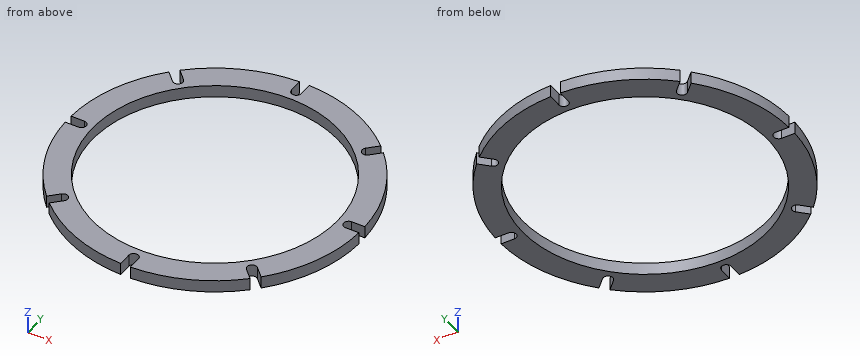
```python
from build123d import *

# Parameters (mm, degrees)
SKETCH1_R           = 121.15
SKETCH1_R_2         = 101.15
BOSS_EXTRUDE1_DEPTH = 10
CUT_EXTRUDE1_DEPTH  = 10
CIRPATTERN1_COUNT   = 8


with BuildPart() as part:
    # Sketch1 → Boss-Extrude1 (new body)
    with BuildSketch(Plane.XY):
        Circle(SKETCH1_R)
        Circle(SKETCH1_R_2, mode=Mode.SUBTRACT)
    extrude(amount=BOSS_EXTRUDE1_DEPTH)

    # Sketch2 → Cut-Extrude1 (cut)
    with BuildSketch(Plane.XY):
        with BuildLine():
            Line((-4, 110.15), (-4, 123.851971246))
            Line((-4, 123.851971246), (4, 123.851971246))
            Line((4, 123.851971246), (4, 110.15))
            ThreePointArc((4, 110.15), (0, 106.15), (-4, 110.15))
        make_face()
    cut_extrude1 = extrude(amount=CUT_EXTRUDE1_DEPTH, mode=Mode.SUBTRACT)

    # CirPattern1: Cut-Extrude1 ×8 about axis
    cirpattern1_axis = Axis((0, 0, 0), (0, 0, 1))
    for i in range(1, CIRPATTERN1_COUNT):
        add(cut_extrude1.rotate(cirpattern1_axis, i * 360 / CIRPATTERN1_COUNT), mode=Mode.SUBTRACT)


solid = part.part
```
Geometry check sheet. Reference: the model listing, model coordinates, mm. Give positions to 0.01 mm unless a question says otherwise; leave off trailing zeros. Write each loop counter-clockwise with the first axis right and the second up, starting at its lowest first coordinate (ties: lowest second). Pieces come first, ordered by that corner, then holes.
1) Material ranges on L1, parallel to Y at x = 0, z = 4.5; L2, parallel to X at y = -77.5, z = 1; L3, parallel to X at y = -82.5, z = 7.5, recorded low to high.
2) Section check A-A, the plane y = 0. Record the boundary of the cut face in (x, z).
3) Gauge pin test, flat ends, axial feed: pin 1 (3 mm diameter, centred on x = -113.5, z = 4, fed in from +Y); pin 2 (4 mm diameter, centred on y = 48, z = 6, fed in from +X); pin 3 (2 mm diameter, centred on x = -9.5, z = 6, fed in from -Y). Record the tip position at first contact, or that the pin passes through.
Computed:
1. L1: y = -106.15 to -101.15, 101.15 to 106.15
1. L2: x = -93.12 to -83.16, -73.91 to -65, 65 to 73.91, 83.16 to 93.12
1. L3: x = -88.72 to -88.16, -76.84 to -58.52, 58.52 to 76.84, 88.16 to 88.72
2. outline: (-106.15, 0) - (-101.15, 0) - (-101.15, 10) - (-106.15, 10) - close; (101.15, 0) - (106.15, 0) - (106.15, 10) - (101.15, 10) - close
3. pin 1: stops at y = 46.19
3. pin 2: stops at x = 112.08
3. pin 3: stops at y = -120.85
